Can you work these out from the drawing? Everything is in mm from the part's minimum corner. Round coordinates to 2 decimals unless told otherwise and drop trailing zeros. Loops run counter-clockwise (first coordinate to the right, second up) from the corner with the lowest first, then second, coordinate; pieces in that order, holes last. Notation, with made-up numbers: M 40,-38.75 L 80,-38.75 A15 ccw 80,-14.75 Z; hole C 84,-15 d5. An arc over 180 degrees is marked long. Use a Markdown table: item, result.
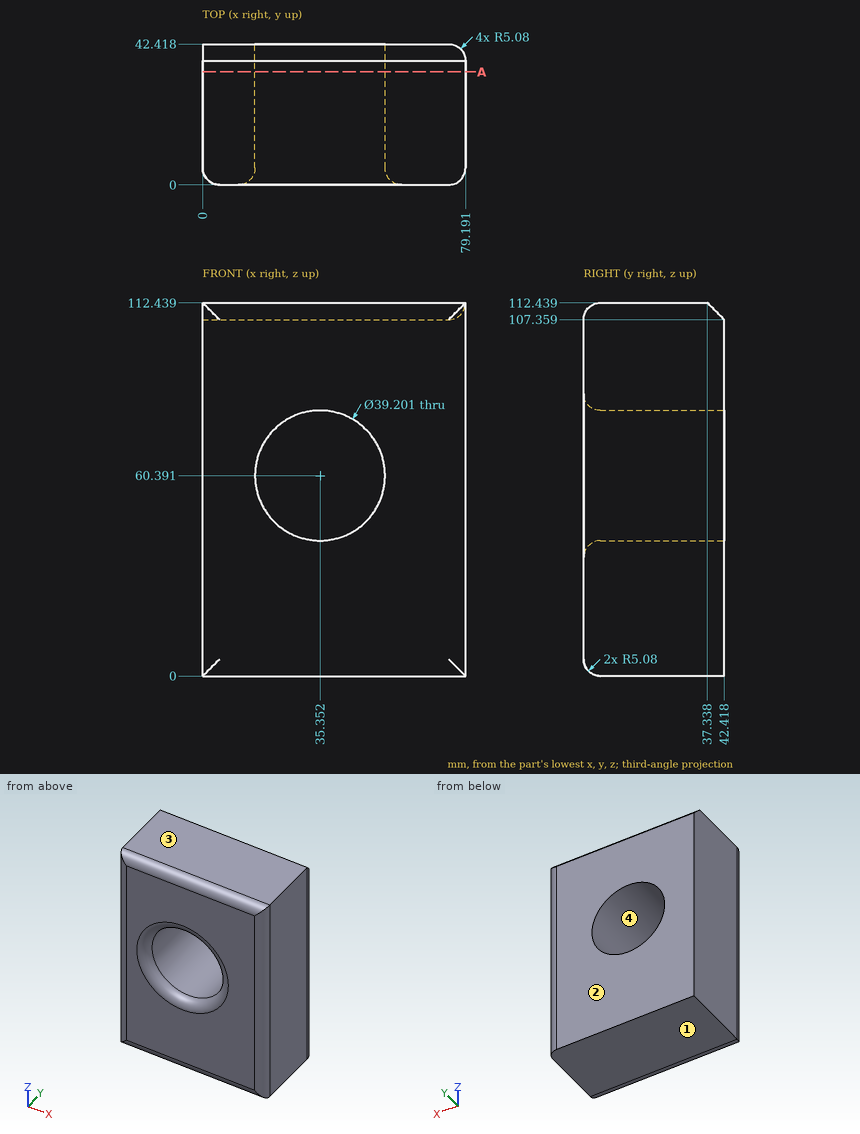
1. We'd pull the mould along Z, two halves only. Please class the marked faces 1, 2, 3 and 4: +Z half, -Z half, draft (parallel to the pull), parting line (faces both ways), or undercut.
Answer sheet:
| item | result |
|---|---|
| face 1 | -Z half |
| face 2 | draft |
| face 3 | +Z half |
| face 4 | undercut |
2. I need wall thicknesses on probe 1 along X at (y, z) = (9.5, 74) (1 decimal); probe 2 along X at (y, z) = (22, 70) (1 decimal); probe 3 along Z at (x, y) = (37, 41) (1 decimal). Which ranges of each line are inside material? Lowest first, please. Write a range as from..to.
Answer sheet:
| item | result |
|---|---|
| probe 1 | 0..21.2, 49.5..79.2 |
| probe 2 | 0..18.3, 52.4..79.2 |
| probe 3 | 0..40.9, 79.9..108.8 |
3. For pin 1 Ø5 at (x, y) = (67.5, 17.5) entering from -Z, with a flat end and sliding along its axis, tell me the tip position at first contact or that it passes through.
Answer sheet:
| item | result |
|---|---|
| pin 1 | z = 0 |
4. Imagine slicing it at A-A, the plane y = 34. Write out the boundary of the cut face in (x, z).
Answer sheet:
| item | result |
|---|---|
| outline | M 0,0 L 79.19,0 L 79.19,112.44 L 0,112.44 Z; hole C 35.35,60.39 d39.2 |
